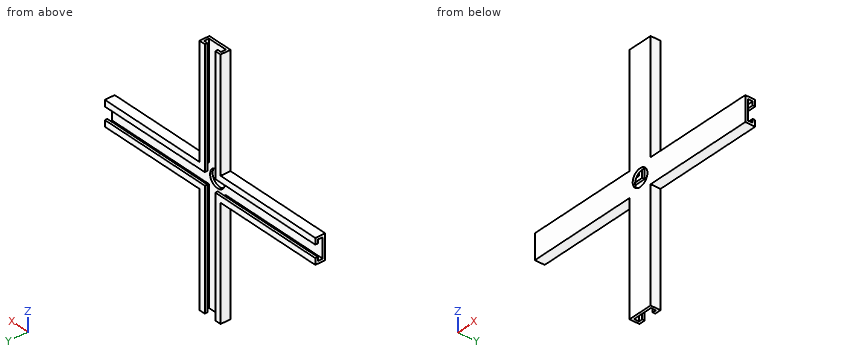
from build123d import *

# Parameters (mm, degrees)
EXTRUDE_1_DEPTH     = 200
EXTRUDE_2_DEPTH     = 100
CUT_EXTRUDE_1_DEPTH = 200
CUT_EXTRUDE_2_DEPTH = 200
CUT_EXTRUDE_3_DEPTH = 15


with BuildPart() as part:
    # 草图1 → 凸台-拉伸1 (new body)
    with BuildSketch(Plane.XY):
        Polygon((0, 0), (10, 0), (10, 8), (5, 8), (5, 6), (8, 6), (8, 2), (0, 2), (-8, 2), (-8, 6), (-5, 6), (-5, 8), (-10, 8), (-10, 0), align=None)
    extrude(amount=EXTRUDE_1_DEPTH)

    # 草图2 → 凸台-拉伸2 (add, symmetric)
    with BuildSketch(Plane(origin=(0, 0, 0), x_dir=(0, 0, -1), z_dir=(1, 0, 0))):
        Polygon((-100, 0), (-90, 0), (-90, 8), (-95, 8), (-95, 6), (-92, 6), (-92, 2), (-100, 2), (-108, 2), (-108, 6), (-105, 6), (-105, 8), (-110, 8), (-110, 0), align=None)
    extrude(amount=EXTRUDE_2_DEPTH, both=True)

    # 草图3 → 切除-拉伸1 (cut)
    with BuildSketch(Plane(origin=(100, 0, 0), x_dir=(0, 0, -1), z_dir=(1, 0, 0))):
        Polygon((-108, 6), (-105, 6), (-105, 8), (-95, 8), (-95, 6), (-92, 6), (-92, 2), (-108, 2), align=None)
    extrude(amount=-CUT_EXTRUDE_1_DEPTH, mode=Mode.SUBTRACT)

    # 草图4 → 切除-拉伸2 (cut)
    with BuildSketch(Plane.XY.offset(200)):
        Polygon((5, 6), (8, 6), (8, 2), (-8, 2), (-8, 6), (-5, 6), (-5, 8), (5, 8), align=None)
    extrude(amount=-CUT_EXTRUDE_2_DEPTH, mode=Mode.SUBTRACT)

    # 草图5 → 切除-拉伸3 (cut)
    with BuildSketch(Plane.XZ):
        with BuildLine():
            ThreePointArc((4.949747468, 104.949747468), (-4.949747468, 104.949747468), (-4.949747468, 95.050252532))
            Line((-4.949747468, 95.050252532), (4.949747468, 104.949747468))
        make_face()
        with BuildLine():
            Line((4.949747468, 104.949747468), (-4.949747468, 95.050252532))
            ThreePointArc((-4.949747468, 95.050252532), (2.678784027, 93.532843272), (7, 100))
            ThreePointArc((7, 100), (6.467156728, 102.678784027), (4.949747468, 104.949747468))
        make_face()
    extrude(amount=-CUT_EXTRUDE_3_DEPTH, mode=Mode.SUBTRACT)


solid = part.part
Verification items for the finished model (mm, model axes). Round coordinates to 2 decimals unless told otherwise and drop trailing zeros. Order: outer loops, then holes, each group sorted by start corner. A loop starts at its lowest first (then second) coordinate and runs counter-clockwise, first axis right, second up. Notation, with made-up numbers: (-2, -7) -> (2, -7) arc R27 ccw to (2, 19) -> close; hole circle Ø2 at (50.5, -31). An arc over 180 degrees is marked (long way). Put each result on its own line as item: value.
1) Section check A-A (y = 3.75). Record the cut outline in (x, z), then the cut area to 3 significant figures.
Final values:
outline: (-100, 90) -> (-10, 90) -> (-10, 0) -> (-8, 0) -> (-8, 92) -> (-100, 92) -> close; (-100, 108) -> (-8, 108) -> (-8, 200) -> (-10, 200) -> (-10, 110) -> (-100, 110) -> close; (8, 0) -> (10, 0) -> (10, 90) -> (100, 90) -> (100, 92) -> (8, 92) -> close; (8, 108) -> (100, 108) -> (100, 110) -> (10, 110) -> (10, 200) -> (8, 200) -> close
area: 1,460 mm^2
2) Depth check by flat-ended pin: pin 1 (2.5 mm diameter, centred on y = 2.5, z = 52, fed in from +X); pin 2 (2 mm diameter, centred on x = -38, y = 5, fed in from -Z); pin 3 (10 mm diameter, centred on x = -3.5, z = 147.5, fed in from -Y); pin 4 (4 mm diameter, centred on x = -59.5, y = 2, fed in from +Z). Enter the tip coordinate at first touch or a pass-through.
Final values:
pin 1: stops at x = 10
pin 2: stops at z = 90
pin 3: stops at y = 0
pin 4: stops at z = 110
3) Section check D-D (x = 74). Record the cut outline in (y, z), then the cut area to 3 significant figures.
Final values:
outline: (0, 90) -> (8, 90) -> (8, 95) -> (6, 95) -> (6, 92) -> (2, 92) -> (2, 108) -> (6, 108) -> (6, 105) -> (8, 105) -> (8, 110) -> (0, 110) -> close
area: 76.0 mm^2
4) Material ranges on line 1 (X direction, y = 7.5, z = 92); line 2 (X direction, y = 5, z = 49); line 3 (Z direction, x = -11.5, y = 7.5), recorded low to high.
Final values:
line 1: x = -100 to -5, 5 to 100
line 2: x = -10 to -8, 8 to 10
line 3: z = 90 to 95, 105 to 110
5) Section check C-C (z = 146). Record the cut outline in (x, y).
Final values:
outline: (-10, 0) -> (10, 0) -> (10, 8) -> (5, 8) -> (5, 6) -> (8, 6) -> (8, 2) -> (-8, 2) -> (-8, 6) -> (-5, 6) -> (-5, 8) -> (-10, 8) -> close
6) Section check B-B (x = 0). Record the cut outline in (y, z).
Final values:
outline: (0, 0) -> (2, 0) -> (2, 93) -> (0, 93) -> close; (0, 107) -> (2, 107) -> (2, 200) -> (0, 200) -> close
